Source: CAD feature listing. Evaluate the final solid. Frame: model axes, mm. A direction names the side the tool comes from. Give positions to 0.01 mm unless a question says otherwise; leave off trailing zeros. Order: outer loops, then holes, each group sorted by start corner. A loop starts at its lowest first (then second) coordinate and runs counter-clockwise, first axis right, second up. Notation, with made-up numbers: M 24.25,5 L 77.25,5 A19 ccw 77.25,23 Z; hole C 46,80 d6. An arc over 180 degrees is marked long. Return JSON: item names as keys, results as strings.
from build123d import *

# Parameters (mm, degrees)
SKETCH1_R           = 2.505
BOSS_EXTRUDE2_DEPTH = 9.5
CUT_EXTRUDE1_REACH  = 12
SKETCH2_R           = 2.005
SKETCH2_R_2         = 2
SKETCH3_W           = 72.995776
SKETCH3_H           = 18.148858384
CUT_EXTRUDE2_DEPTH  = 0.5


with BuildPart() as part:
    # Sketch1 → Boss-Extrude2 (new body)
    with BuildSketch(Plane.XY):
        with BuildLine():
            Line((-11.03, 0), (-28.03, 0))
            Line((-28.03, 0), (-28.03, 10))
            Line((-28.03, 10), (-17.842887818, 10))
            ThreePointArc((-17.842887818, 10), (-14.869374743, 14.045296026), (-11, 17.244380119))
            Line((-11, 17.244380119), (11, 17.244380119))
            ThreePointArc((11, 17.244380119), (14.869374743, 14.045296026), (17.842887818, 10))
            Line((17.842887818, 10), (28.03, 10))
            Line((28.03, 10), (28.03, 0))
            Line((28.03, 0), (11.03, 0))
            ThreePointArc((11.03, 0), (0, 11.03), (-11.03, 0))
        make_face()
        with Locations((11, 11.618950039)):
            Circle(SKETCH1_R, mode=Mode.SUBTRACT)
        with Locations((-11, 11.618950039)):
            Circle(SKETCH1_R, mode=Mode.SUBTRACT)
    extrude(amount=BOSS_EXTRUDE2_DEPTH)

    # Sketch2 → Cut-Extrude1 (cut, up to next)
    with BuildSketch(Plane(origin=(0, 10, 0), x_dir=(1, 0, 0), z_dir=(0, 1, 0)), mode=Mode.PRIVATE) as cut_extrude1_sk1:
        with Locations((22.936443909, -4.75)):
            Circle(SKETCH2_R)
    cut_extrude1_tool1 = extrude(cut_extrude1_sk1.sketch, amount=-CUT_EXTRUDE1_REACH, mode=Mode.PRIVATE) & part.part
    add(cut_extrude1_tool1.solids().sort_by_distance((22.936444, 10, 4.75))[0], mode=Mode.SUBTRACT)
    # Sketch2 → Cut-Extrude1 (cut, up to next)
    with BuildSketch(Plane(origin=(0, 10, 0), x_dir=(1, 0, 0), z_dir=(0, 1, 0)), mode=Mode.PRIVATE) as cut_extrude1_sk2:
        with Locations((-22.936443909, -4.75)):
            Circle(SKETCH2_R_2)
    cut_extrude1_tool2 = extrude(cut_extrude1_sk2.sketch, amount=-CUT_EXTRUDE1_REACH, mode=Mode.PRIVATE) & part.part
    add(cut_extrude1_tool2.solids().sort_by_distance((-22.936444, 10, 4.75))[0], mode=Mode.SUBTRACT)

    # Sketch3 → Cut-Extrude2 (cut)
    with BuildSketch(Plane.XZ):
        with Locations((1.301113009, 1.807163247)):
            Rectangle(SKETCH3_W, SKETCH3_H)
    extrude(amount=-CUT_EXTRUDE2_DEPTH, mode=Mode.SUBTRACT)


solid = part.part
1. Section query C-C (x = -22.5). Return loops of the section in (y, z).
Evaluation:
{"outline": "M 0.5,0 L 10,0 L 10,2.8 L 0.5,2.8 Z; M 0.5,6.7 L 10,6.7 L 10,9.5 L 0.5,9.5 Z"}
2. Draft query along X for faces 1 (the face through (10.457, 9.174, 4.684)), 2 (the face through (23, 10, 7)), 3 (the face through (-9.84, 9.4, 4.68)), 4 (the face through (28.03, 5, 5)). Return one class per face: pulls with the +X half, pulls with the -X half, needs draft (parallel to the pull), parting line crosses it, or undercut.
Evaluation:
{"face 1": "undercut", "face 2": "needs draft", "face 3": "undercut", "face 4": "pulls with the +X half"}
3. First-contact query: pin 1 (3 mm diameter, centred on x = 24.5, z = 3, fed in from +Y); pin 2 (4 mm diameter, centred on x = -3, y = 8, fed in from +Z); pin 3 (2 mm diameter, centred on x = 4, z = 5.5, fed in from -Y); pin 4 (1 mm diameter, centred on y = 13, z = 5.5, fed in from -X). Flat tips, straight axial feed; report the tip coordinate or a pass-through.
Evaluation:
{"pin 1": "stops at y = 10", "pin 2": "passes through", "pin 3": "stops at y = 9.83", "pin 4": "stops at x = -16.19"}
4. Section query D-D (y = 13). Return loops of the section in (x, z), then the cut area to 3 significant figures.
Evaluation:
{"outline": "M -15.79,0 L -13.09,0 L -13.09,9.5 L -15.79,9.5 Z; M -8.91,0 L 8.91,0 L 8.91,9.5 L -8.91,9.5 Z; M 13.09,0 L 15.79,0 L 15.79,9.5 L 13.09,9.5 Z", "area": "221 mm^2"}
5. Ray query, probe 1 along X at (y, z) = (13, 6.5); probe 2 along Y at (x, z) = (26.5, 1.5); probe 3 along X at (y, z) = (4.25, 7.5). Return the intervals inside material, ascending.
Evaluation:
{"probe 1": "x = -15.79 to -13.09, -8.91 to 8.91, 13.09 to 15.79", "probe 2": "y = 0.5 to 10", "probe 3": "x = -28.03 to -10.18, 10.18 to 28.03"}
6. Set-up query: faces 5 (the face through (14.82, 14.1, 4.68)), 6 (the face through (-23, 10, 7)). Return all of +Z, -Z, +X, -X, +Y, -Y with unobstructed straight access to the full face (end or side cutting, diameter ignored); none if empty.
Evaluation:
{"face 5": "+Z, -Z, +X, +Y", "face 6": "+Z, -Z, -X, +Y"}
7. Section query B-B (y = 5). Return loops of the section in (x, z) (3 decimals), then the cut area to 3 significant figures.
Evaluation:
{"outline": "M -28.03,0 L -9.832,0 L -9.832,9.5 L -28.03,9.5 Z; M 9.832,0 L 28.03,0 L 28.03,9.5 L 9.832,9.5 Z; hole C -22.936,4.75 d4; hole C 22.936,4.75 d4.01", "area": "321 mm^2"}
8. Section query A-A (z = 3.5). Return loops of the section in (x, y) (3 decimals).
Evaluation:
{"outline": "M -28.03,0.5 L -24.498,0.5 L -24.498,10 L -28.03,10 Z; M -21.375,0.5 L -11.019,0.5 A11.03 cw 11.019,0.5 L 21.369,0.5 L 21.369,10 L 17.843,10 A20.454 ccw 11,17.244 L -11,17.244 A20.454 ccw -17.843,10 L -21.375,10 Z; M 24.504,0.5 L 28.03,0.5 L 28.03,10 L 24.504,10 Z; hole C -11,11.619 d5.01; hole C 11,11.619 d5.01"}
